Source: three-view drawing plus pictorial views. Frame: mm from the lowest corner of the part. A direction names the side the tool comes from. Round coordinates to 2 decimals unless told otherwise and drop trailing zeros. Order: outer loops, then holes, each group sorted by start corner. A loop starts at its lowest first (then second) coordinate and runs counter-clockwise, first axis right, second up. Notation, with made-up numbers: (23, 29) -> (59, 29) arc R10 ccw to (59, 38) -> close; hole circle Ø1 at (41.25, -9). An arc over 180 degrees is marked (long way). Answer as CSV lines item,"result". Start each with the question number.
1) Access query for the marked faces 4 and 5. Directions: +Z, -Z, +X, -X, +Y, -Y. A direction counts if a zero-diameter tool reaches every point of the face in a straight line with its end or side. Return the directions, or none.
2) Line query: L1, parallel to Y at x = 0.4, z = 3.5 (1 decimal); L2, parallel to Z at x = 2.75, y = 13; L3, parallel to Y at x = 3.2, z = 1.55 (1 decimal). Output: solid intervals per line, ascending.
3) Mould query, pull axis Z, two halves, no side actions, for the marked faces 1, 2 and 3. Classes: +Z half, -Z half, draft (parallel to the pull), parting line (faces both ways), or undercut.
4) Section query B-B, the plane y = 9.75. Output: boundary loops of the cut face in (x, z).
5) First-contact query: P1, Ø1, axis at x = 5, y = 2, coming from the -Z side; P2, Ø0.8, axis at y = 15, z = 2.5, coming from the +X side; P3, Ø1.4, axis at x = 3.5, z = 2.5, coming from the +Y side (1 decimal); P4, Ø1.5, axis at x = 5, y = 11.5, coming from the +Z side. Flat tips, straight axial feed; report the tip coordinate or a pass-through.
6) Section query A-A, the plane y = 15. Output: boundary loops of the cut face in (x, z), and give its area (3 significant figures).
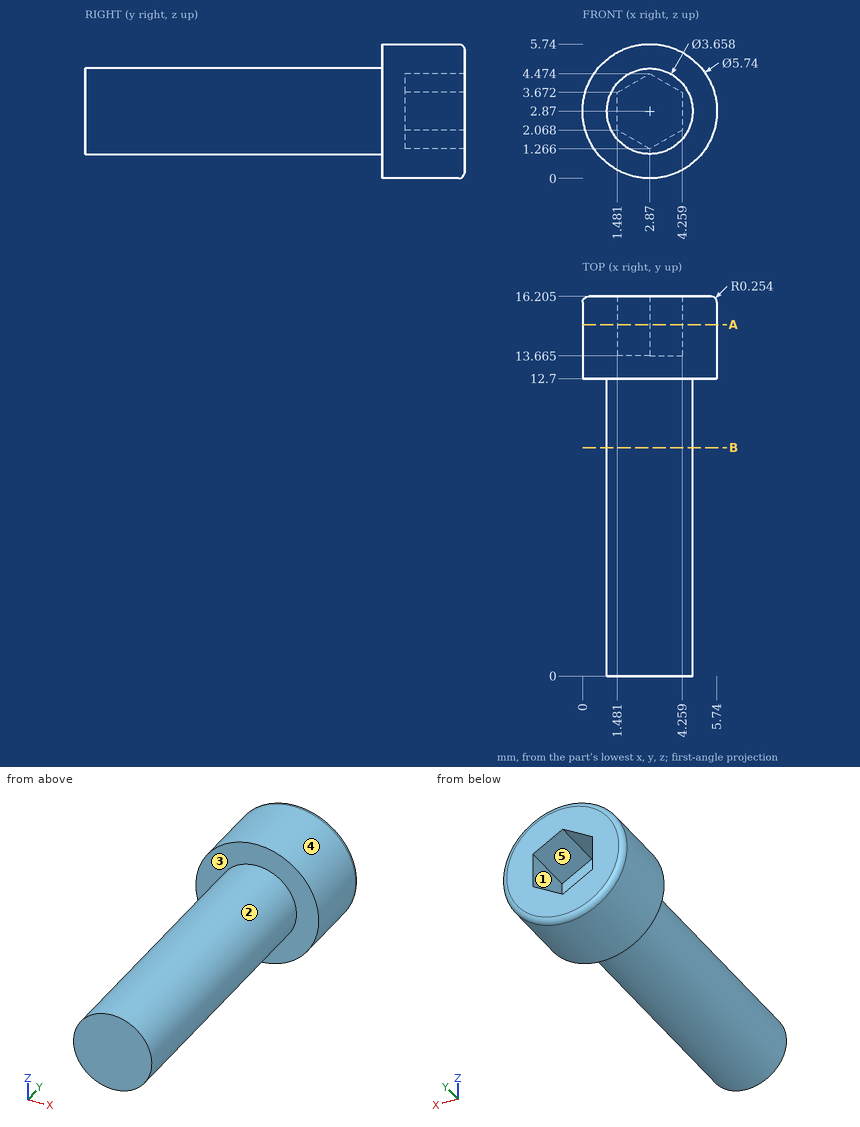
Findings:
1,face 4,"+Y, -Y"
1,face 5,"+Y"
2,L1,"y = 12.7 to 16.2"
2,L2,"z = 0 to 5.74"
2,L3,"y = 0 to 13.7"
3,face 1,"undercut"
3,face 2,"parting line"
3,face 3,"draft"
4,outline,"circle Ø3.66 at (2.87, 2.87)"
5,P1,"stops at z = 2.04"
5,P2,"stops at x = 5.74"
5,P3,"stops at y = 13.7"
5,P4,"stops at z = 4.07"
6,outline,"circle Ø5.74 at (2.87, 2.87); hole (1.48, 2.07) -> (2.87, 1.27) -> (4.26, 2.07) -> (4.26, 3.67) -> (2.87, 4.47) -> (1.48, 3.67) -> close"
6,area,"19.2 mm^2"
